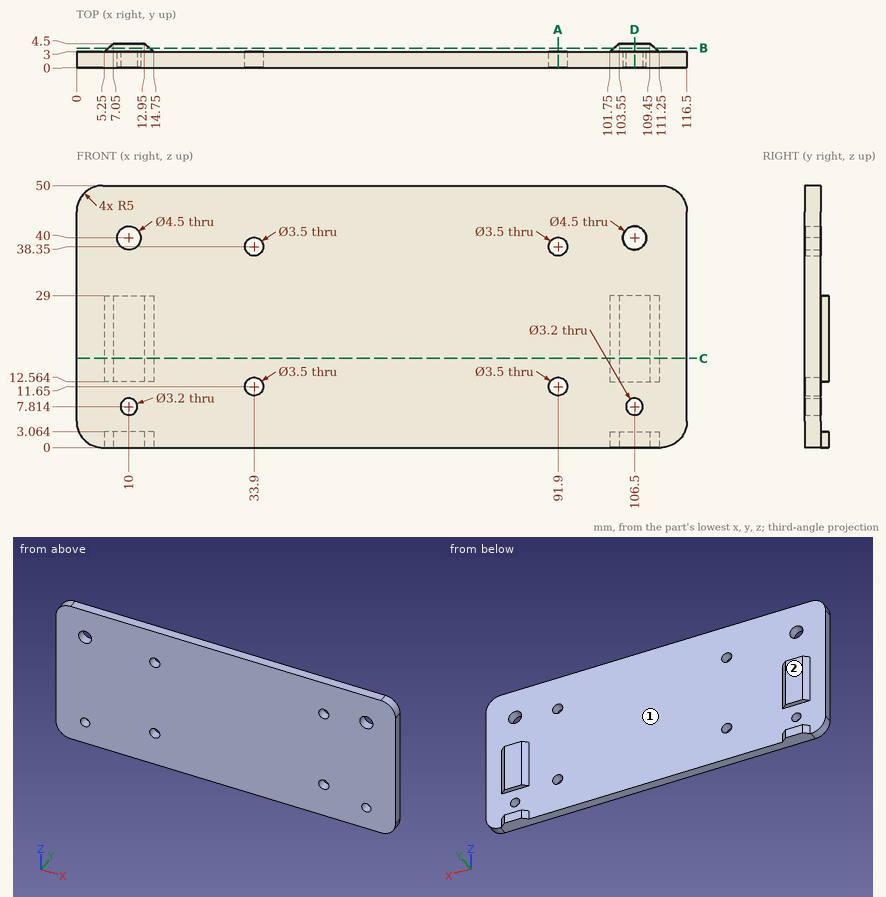
Input: dimensioned drawing with shaded views. Units: mm. Origin: part minimum x, y, z. Round coordinates to 2 decimals unless told otherwise and drop trailing zeros. Loops run counter-clockwise (first coordinate to the right, second up) from the corner with the lowest first, then second, coordinate; pieces in that order, holes last. Notation, with made-up numbers: (37.5, 75.25) -> (70.5, 75.25) arc R5 ccw to (70.5, 80.25) -> close; hole circle Ø6 at (-14, 68). An arc over 180 degrees is marked (long way). Answer as a JSON object with one key per item and string values. Group by question number.
1) Section query D-D on x = 106.5. Output: boundary loops of the cut face in (y, z).
2) Draft query along X for the marked faces 1 and 2. Return one class per face: +X half, -X half, draft (parallel to the pull), parting line (faces both ways), or undercut.
3) Pin query (flat end, axial travel): pin 1 (3 mm diameter, centred on x = 44.5, z = 34, fed in from +Y); pin 2 (0.8 mm diameter, centred on x = 107.5, y = 4, fed in from +Z); pin 3 (3 mm diameter, centred on x = 91.9, z = 11.65, fed in from +Y). Return the tip coordinate at first contact, or that it passes through.
4) Section query B-B on y = 3.7. Output: boundary loops of the cut face in (x, z), plus the area to 3 significant figures.
5) Section query C-C on z = 17. Output: boundary loops of the cut face in (x, y), plus the area to 3 significant figures.
6) Ray query, L1, parallel to Z at x = 91.9, y = 0.85; L2, parallel to Z at x = 10, y = 0.7; L3, parallel to Y at x = 48, z = 25.5. Return the intervals inside material, ascending.
7) Section query A-A on x = 91.9. Output: boundary loops of the cut face in (y, z).
Reply:
{
 "1": {"outline": "(0, 0) -> (4.5, 0) -> (4.5, 3.06) -> (3, 3.06) -> (3, 6.21) -> (0, 6.21) -> close; (0, 9.41) -> (3, 9.41) -> (3, 12.56) -> (4.5, 12.56) -> (4.5, 29) -> (3, 29) -> (3, 37.75) -> (0, 37.75) -> close; (0, 42.25) -> (3, 42.25) -> (3, 50) -> (0, 50) -> close"},
 "2": {"face 1": "undercut", "face 2": "draft"},
 "3": {"pin 1": "stops at y = 3", "pin 2": "stops at z = 29", "pin 3": "passes through"},
 "4": {"outline": "(6.09, 0) -> (13.91, 0) -> (13.91, 3.06) -> (6.09, 3.06) -> close; (6.09, 12.56) -> (13.91, 12.56) -> (13.91, 29) -> (6.09, 29) -> close; (102.59, 0) -> (110.41, 0) -> (110.41, 3.06) -> (102.59, 3.06) -> close; (102.59, 12.56) -> (110.41, 12.56) -> (110.41, 29) -> (102.59, 29) -> close", "area": "305 mm2"},
 "5": {"outline": "(0, 0) -> (116.5, 0) -> (116.5, 3) -> (111.25, 3) -> (109.45, 4.5) -> (103.55, 4.5) -> (101.75, 3) -> (14.75, 3) -> (12.95, 4.5) -> (7.05, 4.5) -> (5.25, 3) -> (0, 3) -> close", "area": "373 mm2"},
 "6": {"L1": "z = 0 to 9.9, 13.4 to 36.6, 40.1 to 50", "L2": "z = 0 to 6.21, 9.41 to 37.75, 42.25 to 50", "L3": "y = 0 to 3"},
 "7": {"outline": "(0, 0) -> (3, 0) -> (3, 9.9) -> (0, 9.9) -> close; (0, 13.4) -> (3, 13.4) -> (3, 36.6) -> (0, 36.6) -> close; (0, 40.1) -> (3, 40.1) -> (3, 50) -> (0, 50) -> close"}
}
